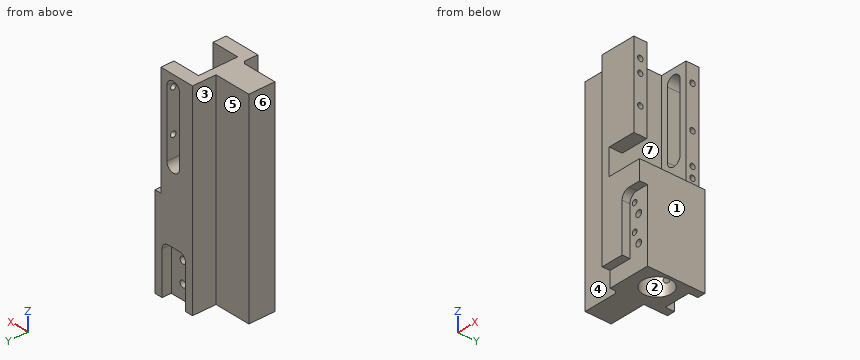
from build123d import *

# Parameters (mm, degrees)
EXTRUDE_1_DEPTH          = 155
EXTRUDE_2_REACH          = 173.901
SKETCH_2_W               = 32
SKETCH_2_H               = 70
CUT_EXTRUDE_1_DEPTH      = 172.901134377
CUT_EXTRUDE_1_DEPTH_BACK = 7
CUT_EXTRUDE_2_REACH      = 173.901
CUT_EXTRUDE_3_REACH      = 114.916
SKETCH_5_R               = 6
CUT_EXTRUDE_START        = -70
SKETCH_6_R               = 10.5
CUT_EXTRUDE_4_DEPTH      = 55
M24X2_0_1_D              = 22
M24X2_0_1_DEPTH          = 15
M24X2_0_1_TIP            = 6.609466809
HOLE_WIZARD_M6_1_REACH   = 171.997
HOLE_WIZARD_M6_1_BORE_R  = 2.5
HOLE_WIZARD_M5_1_D       = 4.2
HOLE_WIZARD_M5_1_DEPTH   = 5
SKETCH_15_W              = 20
SKETCH_15_H              = 10
CUT_EXTRUDE_5_DEPTH      = 21
HOLE_WIZARD_M5_2_D       = 4.2
HOLE_WIZARD_M5_2_DEPTH   = 13
HOLE_WIZARD_M5_2_TIP     = 1.2618073
F_4_0MM_1_D              = 4
F_4_0MM_1_DEPTH          = 12
F_4_0MM_1_TIP            = 1.201721238
CUT_EXTRUDE_7_DEPTH      = 172.901134467
CUT_EXTRUDE_7_DEPTH_BACK = 6
F_4_0MM_2_D              = 4
F_4_0MM_2_DEPTH          = 10
F_4_0MM_2_TIP            = 1.201721238
HOLE_WIZARD_M6_2_D       = 5
HOLE_WIZARD_M6_2_DEPTH   = 12
HOLE_WIZARD_M6_2_TIP     = 1.502151548
CHAMFER_1_SIZE           = 2


with BuildPart() as part:
    # 草图1 → 凸台-拉伸1 (new body)
    with BuildSketch(Plane.XY):
        Polygon((0, 0), (-27, 0), (-27, 12), (-55, 12), (-55, 32), (-27, 32), (-27, 50), (0, 50), (0, 40), (-21, 40), (-21, 10), (0, 10), align=None)
    extrude(amount=-EXTRUDE_1_DEPTH)

    # 凸台-拉伸2: up to this face of the body (flat: up to its plane)
    extrude_2_end = Plane(part.part.faces().sort_by_distance((-13.5, 50, -77.5))[0])
    # 草图2 → 凸台-拉伸2 (add, up to the picked face)
    with BuildSketch(Plane(origin=(0, 0, 0), x_dir=(1, 0, 0), z_dir=(0, 1, 0)), mode=Mode.PRIVATE) as extrude_2_sk1:
        with Locations((-11, 120)):
            Rectangle(SKETCH_2_W, SKETCH_2_H)
    extrude_2_tool1 = split(extrude(extrude_2_sk1.sketch, amount=EXTRUDE_2_REACH, mode=Mode.PRIVATE), bisect_by=extrude_2_end, keep=Keep.BOTH, mode=Mode.PRIVATE)
    add(extrude_2_tool1.solids().sort_by(Axis((-11, 0, -120), (0, 1, 0)))[0])

    # 草图3 → 切除-拉伸1 (cut, two sides: drawn at the far end of the back side and taken through both)
    with BuildSketch(Plane(origin=(0, 50, 0), x_dir=(1, 0, 0), z_dir=(0, 1, 0)).offset(-CUT_EXTRUDE_1_DEPTH_BACK)):
        with BuildLine():
            Line((-6, 117), (-16, 117))
            ThreePointArc((-16, 117), (-19.535533906, 118.464466094), (-21, 122))
            Line((-21, 122), (-21, 155))
            Line((-21, 155), (-1, 155))
            Line((-1, 155), (-1, 122))
            ThreePointArc((-1, 122), (-2.464466094, 118.464466094), (-6, 117))
        make_face()
    extrude(amount=CUT_EXTRUDE_1_DEPTH + CUT_EXTRUDE_1_DEPTH_BACK, mode=Mode.SUBTRACT)

    # 草图4 → 切除-拉伸2 (cut, up to next)
    with BuildSketch(Plane(origin=(0, 50, 0), x_dir=(1, 0, 0), z_dir=(0, 1, 0)), mode=Mode.PRIVATE) as cut_extrude_2_sk1:
        with BuildLine():
            Line((-16, 10), (-16, 61))
            ThreePointArc((-16, 61), (-10.5, 66.5), (-5, 61))
            Line((-5, 61), (-5, 10))
            ThreePointArc((-5, 10), (-10.5, 4.5), (-16, 10))
        make_face()
    cut_extrude_2_tool1 = extrude(cut_extrude_2_sk1.sketch, amount=-CUT_EXTRUDE_2_REACH, mode=Mode.PRIVATE) & part.part
    add(cut_extrude_2_tool1.solids().sort_by_distance((-10.5, 50, -35.5))[0], mode=Mode.SUBTRACT)

    # 草图5 → 切除-拉伸3 (cut, up to next)
    with BuildSketch(Plane.XY.offset(-85), mode=Mode.PRIVATE) as cut_extrude_3_sk1:
        with Locations((-8, 25)):
            Circle(SKETCH_5_R)
    cut_extrude_3_tool1 = extrude(cut_extrude_3_sk1.sketch, amount=-CUT_EXTRUDE_3_REACH, mode=Mode.PRIVATE) & part.part
    add(cut_extrude_3_tool1.solids().sort_by_distance((-8, 25, -85))[0], mode=Mode.SUBTRACT)

    # 草图6 → 切除-拉伸4 (cut)
    with BuildSketch(Plane.XY.offset(-85).offset(CUT_EXTRUDE_START)):
        with Locations(Location((-8, 25, 0), (0, 0, 180))):
            Circle(SKETCH_6_R)
    extrude(amount=CUT_EXTRUDE_4_DEPTH, mode=Mode.SUBTRACT)

    # M24x2.0 螺纹孔1
    with Locations(Plane(origin=(0, 0, -155), x_dir=(-1, 0, 0), z_dir=(0, 0, -1))):
        with Locations((8, 25)):
            Hole(M24X2_0_1_D / 2, depth=M24X2_0_1_DEPTH)
            with Locations((0, 0, -(M24X2_0_1_DEPTH + M24X2_0_1_TIP / 2))):  # 118° drill point
                Cone(0, M24X2_0_1_D / 2, M24X2_0_1_TIP, mode=Mode.SUBTRACT)

    # M6 螺纹孔1 bore → M6 螺纹孔1 (cut, up to next)
    with BuildSketch(Plane(origin=(0, 43, 0), x_dir=(1, 0, 0), z_dir=(0, 1, 0)), mode=Mode.PRIVATE) as hole_wizard_m6_1_sk1:
        with Locations((-11, 144)):
            Circle(HOLE_WIZARD_M6_1_BORE_R)
    hole_wizard_m6_1_tool1 = extrude(hole_wizard_m6_1_sk1.sketch, amount=-HOLE_WIZARD_M6_1_REACH, mode=Mode.PRIVATE) & part.part
    # M6 螺纹孔1 bore → M6 螺纹孔1 (cut, up to next)
    with BuildSketch(Plane(origin=(0, 43, 0), x_dir=(1, 0, 0), z_dir=(0, 1, 0)), mode=Mode.PRIVATE) as hole_wizard_m6_1_sk2:
        with Locations((-11, 128)):
            Circle(HOLE_WIZARD_M6_1_BORE_R)
    hole_wizard_m6_1_tool2 = extrude(hole_wizard_m6_1_sk2.sketch, amount=-HOLE_WIZARD_M6_1_REACH, mode=Mode.PRIVATE) & part.part
    add(hole_wizard_m6_1_tool1.solids().sort_by_distance((-11, 43, -144))[0], mode=Mode.SUBTRACT)
    add(hole_wizard_m6_1_tool2.solids().sort_by_distance((-11, 43, -128))[0], mode=Mode.SUBTRACT)

    # M5 螺纹孔1
    with Locations(Plane(origin=(0, 0, 0), x_dir=(0, 0, -1), z_dir=(1, 0, 0))):
        with Locations((13, 45), (45, 45)):
            Hole(HOLE_WIZARD_M5_1_D / 2, depth=HOLE_WIZARD_M5_1_DEPTH)

    # 草图15 → 切除-拉伸5 (cut)
    with BuildSketch(Plane(origin=(0, 0, 0), x_dir=(0, 0, -1), z_dir=(1, 0, 0))):
        with Locations((75, 5)):
            Rectangle(SKETCH_15_W, SKETCH_15_H)
    extrude(amount=-CUT_EXTRUDE_5_DEPTH, mode=Mode.SUBTRACT)

    # M5 螺纹孔2
    with Locations(Plane(origin=(0, 0, 0), x_dir=(0, 0, -1), z_dir=(1, 0, 0))):
        with Locations((13, 5), (45, 5), (77, 45)):
            Hole(HOLE_WIZARD_M5_2_D / 2, depth=HOLE_WIZARD_M5_2_DEPTH)
            with Locations((0, 0, -(HOLE_WIZARD_M5_2_DEPTH + HOLE_WIZARD_M5_2_TIP / 2))):  # 118° drill point
                Cone(0, HOLE_WIZARD_M5_2_D / 2, HOLE_WIZARD_M5_2_TIP, mode=Mode.SUBTRACT)

    # Ø4.0mm 暗销孔1
    with Locations(Plane(origin=(0, 0, 0), x_dir=(0, 0, -1), z_dir=(1, 0, 0))):
        with Locations((23, 5), (69, 45)):
            Hole(F_4_0MM_1_D / 2, depth=F_4_0MM_1_DEPTH)
            with Locations((0, 0, -(F_4_0MM_1_DEPTH + F_4_0MM_1_TIP / 2))):  # 118° drill point
                Cone(0, F_4_0MM_1_D / 2, F_4_0MM_1_TIP, mode=Mode.SUBTRACT)

    # 草图22 → 切除-拉伸7 (cut, two sides: drawn at the far end of the back side and taken through both)
    with BuildSketch(Plane.XZ.offset(-CUT_EXTRUDE_7_DEPTH_BACK)):
        with BuildLine():
            Line((308.073369653, -100), (5, -100))
            Line((5, -100), (-4, -100))
            ThreePointArc((-4, -100), (-8.242640687, -101.757359313), (-10, -106))
            Line((-10, -106), (-10, -143))
            Line((-10, -143), (-27, -143))
            Line((-27, -143), (-330.073369653, -143))
            Line((-330.073369653, -143), (-289.322022823, -747.775327956))
            Line((-289.322022823, -747.775327956), (348.824716484, -704.775327956))
            Line((348.824716484, -704.775327956), (308.073369653, -100))
        make_face()
    extrude(amount=CUT_EXTRUDE_7_DEPTH + CUT_EXTRUDE_7_DEPTH_BACK, mode=Mode.SUBTRACT)

    # Ø4.0mm 暗销孔2
    with Locations(Plane(origin=(0, 6, 0), x_dir=(-1, 0, 0), z_dir=(0, -1, 0))):
        with Locations((6, 127), (6, 107)):
            Hole(F_4_0MM_2_D / 2, depth=F_4_0MM_2_DEPTH)
            with Locations((0, 0, -(F_4_0MM_2_DEPTH + F_4_0MM_2_TIP / 2))):  # 118° drill point
                Cone(0, F_4_0MM_2_D / 2, F_4_0MM_2_TIP, mode=Mode.SUBTRACT)

    # M6 螺纹孔2
    with Locations(Plane(origin=(0, 6, 0), x_dir=(-1, 0, 0), z_dir=(0, -1, 0))):
        with Locations((2.5, 136), (2.5, 116)):
            Hole(HOLE_WIZARD_M6_2_D / 2, depth=HOLE_WIZARD_M6_2_DEPTH)
            with Locations((0, 0, -(HOLE_WIZARD_M6_2_DEPTH + HOLE_WIZARD_M6_2_TIP / 2))):  # 118° drill point
                Cone(0, HOLE_WIZARD_M6_2_D / 2, HOLE_WIZARD_M6_2_TIP, mode=Mode.SUBTRACT)

    # 倒角1
    chamfer_1_edges = [part.edges().sort_by_distance(p)[0] for p in [
        (-27, 12, -77.5),
    ]]
    chamfer(chamfer_1_edges, length=CHAMFER_1_SIZE)


solid = part.part
Could you check a few things on this model? Use its own coordinates, in mm. Face numbers are marked on the shaded views. A direction names the side the tool comes from. Give positions to 0.01 mm unless a question says otherwise; leave off trailing zeros. Order: outer loops, then holes, each group sorted by start corner. A loop starts at its lowest first (then second) coordinate and runs counter-clockwise, first axis right, second up. Notation, with made-up numbers: (-33.5, 42.5) - (3.5, 42.5) arc R36 cw to (3.5, 76.5) - close; hole circle Ø10 at (76.5, 12.25). An arc over 180 degrees is marked (long way). One line per item, written item: value. Start each with the question number.
1. If I drill on probe 1 along Y at (x, z) = (-8, -93.5); probe 2 along Z at (x, y) = (-3.25, 5); probe 3 along X at (y, z) = (41.5, -19.5), over which ranges is the centre line in solid material (lowest first)?
2. Imagine slicing it at B-B on x = -33.5. List the corners of the cut face in (y, z) for me.
3. Imagine slicing it at A-A on y = 41.5. List the corners of the cut face in (x, z) for me.
4. Thinking about a two-plate mould opening in Y: for the marked faces 4, 5, 6 and 7, which applies, +Y half, -Y half, draft (parallel to the pull), parting line (faces both ways), or undercut?
5. For the marked faces 1, 2 and 3, which set-ups out of +Z, -Z, +X, -X, +Y, -Y let a thin tool reach every point of the face, with its end or its side?
6. For P1, Ø1.5, axis at x = -33.5, z = -112.5, coming from the -Y side; P2, Ø11, axis at y = 47.5, z = -31, coming from the -X side; P3, Ø8, axis at x = -13.5, y = 40.5, coming from the +Z side; P4, Ø6, axis at x = -2.5, z = -136, coming from the -Y side, each with a flat end and sliding along its axis, tell me the tip position at first contact or that it passes through.
Values:
1. probe 1: 0 to 19, 31 to 50
1. probe 2: -100 to -85, -65 to -47.1, -42.9 to -25, -21 to -15.1, -10.9 to 0
1. probe 3: -27 to -16, -5 to 0
2. outline: (12, -155) - (32, -155) - (32, 0) - (12, 0) - close
3. outline: (-27, -155) - (5, -155) - (5, -85) - (0, -85) - (0, 0) - (-27, 0) - close; hole (-16, -61) arc R5.5 ccw to (-5, -61) - (-5, -10) arc R5.5 ccw to (-16, -10) - close; hole circle Ø5 at (-11, -144); hole circle Ø5 at (-11, -128)
4. face 4: -Y half
4. face 5: +Y half
4. face 6: draft
4. face 7: undercut
5. face 1: +Z, -Z, +X, +Y, -Y
5. face 2: -Z
5. face 3: +Z, -Z, -X, +Y
6. P1: y = 12
6. P2: x = -27
6. P3: z = 0
6. P4: y = 6
